from build123d import *

# Parameters (mm, degrees)
SKETCH2_R           = 3
SKETCH2_R_2         = 2
BOSS_EXTRUDE1_DEPTH = 6
SCALE1_SCALE        = 0.5


with BuildPart() as part:
    # Sketch2 → Boss-Extrude1 (new body)
    with BuildSketch(Plane.XY):
        with BuildLine():
            Line((6, 75), (6, -75))
            ThreePointArc((6, -75), (0, -81), (-6, -75))
            Line((-6, -75), (-6, 75))
            ThreePointArc((-6, 75), (0, 81), (6, 75))
        make_face()
        with Locations((0, 75)):
            Circle(SKETCH2_R, mode=Mode.SUBTRACT)
        with Locations((0, 25)):
            Circle(SKETCH2_R, mode=Mode.SUBTRACT)
        with Locations((0, -75)):
            Circle(SKETCH2_R_2, mode=Mode.SUBTRACT)
    extrude(amount=-BOSS_EXTRUDE1_DEPTH)


with BuildPart() as part_1:
    # Scale1: scaled about (0, -1.022220005, -3)
    add(part.part.scale(SCALE1_SCALE).moved(Location((0, -0.511110003, -1.5))))


solid = part_1.part
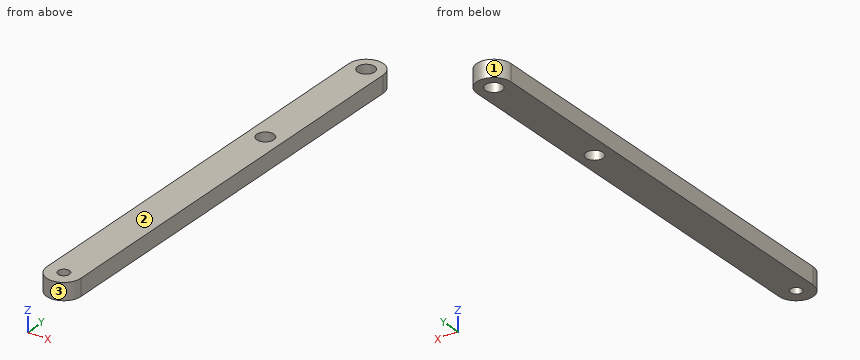
Geometry: final body of the model. Coordinates: model frame, mm. Face numbers are marked on the shaded views. Give positions to 0.01 mm unless a question says otherwise; leave off trailing zeros. Write each loop counter-clockwise with the first axis right and the second up, starting at its lowest first coordinate (ties: lowest second). Pieces come first, ordered by that corner, then holes. Notation, with made-up numbers: (88.5, 12.5) -> (140.5, 12.5) arc R26 ccw to (140.5, 49.5) -> close; hole circle Ø3 at (75, -30.5). An arc over 180 degrees is marked (long way). Answer in a Markdown table with one row per item.
(1) Pin query (flat end, axial travel): pin 1 (1.8 mm diameter, centred on x = 0, y = -38.01, fed in from +Z). Return the tip coordinate at first contact, or that it passes through.
Answers below:
| item | result |
|---|---|
| pin 1 | through |
(2) Draft query along Y for the marked faces 1, 2 and 3. Return one class per face: +Y half, -Y half, draft (parallel to the pull), parting line (faces both ways), or undercut.
Answers below:
| item | result |
|---|---|
| face 1 | +Y half |
| face 2 | draft |
| face 3 | -Y half |
(3) Ray query, line 1 along Y through (x, z) = (0, -3.15); line 2 along Y through (x, z) = (-0.45, -3.05); line 3 along Y through (x, z) = (1.1, -1.65). Return the intervals inside material, ascending. Write a range as [from, to].
Answers below:
| item | result |
|---|---|
| line 1 | [-41.01, -39.01], [-37.01, 10.49], [13.49, 35.49], [38.49, 39.99] |
| line 2 | [-40.98, -38.9], [-37.12, 10.56], [13.42, 35.56], [38.42, 39.95] |
| line 3 | [-40.8, 10.97], [13.01, 35.97], [38.01, 39.78] |
(4) Section query A-A on x = 0. Return loops of the section in (y, z), then the cut area to 3 significant figures.
Answers below:
| item | result |
|---|---|
| outline | (-41.01, -4.5) -> (-39.01, -4.5) -> (-39.01, -1.5) -> (-41.01, -1.5) -> close; (-37.01, -4.5) -> (10.49, -4.5) -> (10.49, -1.5) -> (-37.01, -1.5) -> close; (13.49, -4.5) -> (35.49, -4.5) -> (35.49, -1.5) -> (13.49, -1.5) -> close; (38.49, -4.5) -> (39.99, -4.5) -> (39.99, -1.5) -> (38.49, -1.5) -> close |
| area | 219 mm^2 |
(5) Section query B-B on z = -2.3. Return loops of the section in (x, y).
Answers below:
| item | result |
|---|---|
| outline | (-3, -38.01) arc R3 ccw to (3, -38.01) -> (3, 36.99) arc R3 ccw to (-3, 36.99) -> close; hole circle Ø3 at (0, 11.99); hole circle Ø3 at (0, 36.99); hole circle Ø2 at (0, -38.01) |
